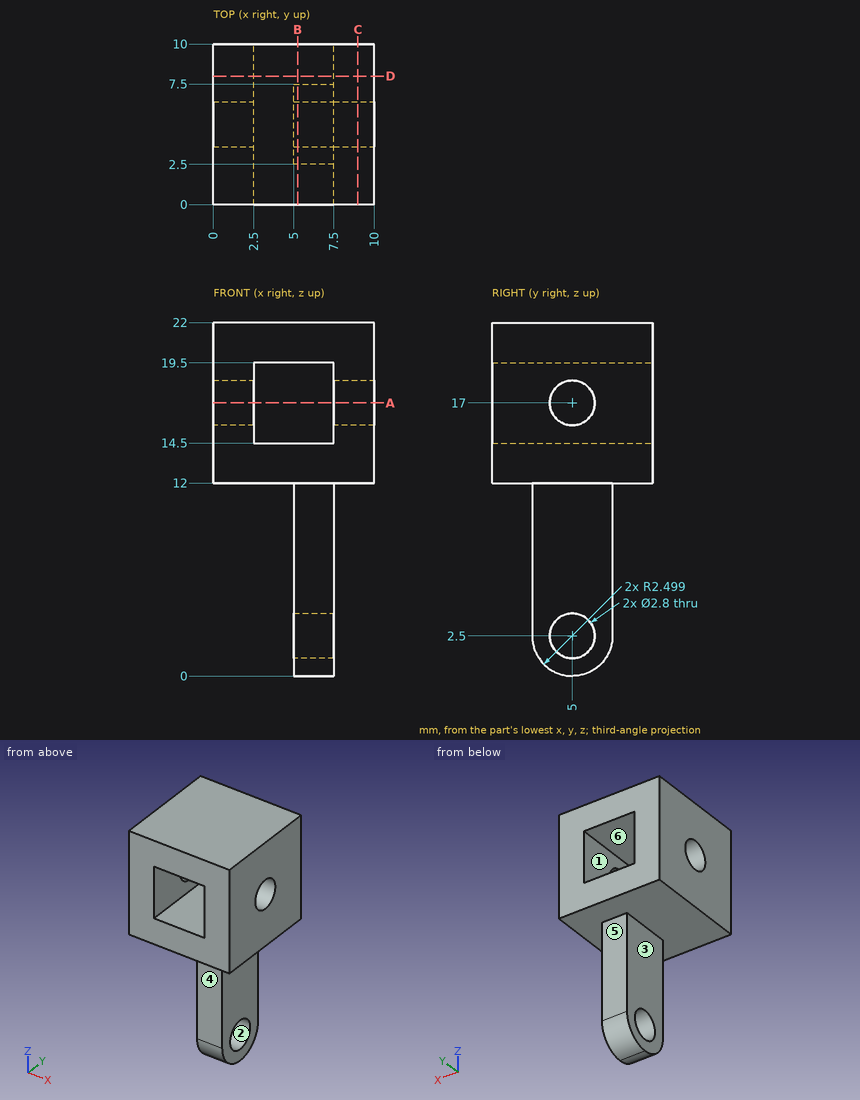
Geometry: see drawing. Coordinates: mm, zero at the bounding-box minimum. A direction names the side the tool comes from. Coordinates: 2 decimals unless noted, no trailing zeros. Loops run counter-clockwise (first coordinate to the right, second up) from the corner with the lowest first, then second, coordinate; pieces in that order, holes last.
(1) Section C-C on x = 9. Return the cut outline in (y, z).
(2) Section D-D on y = 8. Return the cut outline in (x, z).
(3) Material intervals for probe 1 along Y at (x, z) = (1.3, 17); probe 2 along Z at (x, y) = (4, 6.5); probe 3 along X at (y, z) = (5, 15.25), sorted ascending.
(4) Pull-direction query (X, two-part tool) for the marked faces 1, 2 and 3; classes: released by +X, released by -X, zero draft, split by the parting line, or undercut.
(5) Set-up query: the marked faces 4, 5 and 6. Return all of +Z, -Z, +X, -X, +Y, -Y with unobstructed straight access to the full face (end or side cutting, diameter ignored); none if empty.
(6) Section B-B on x = 5.25. Count the separate pieces of the cut face and the enclosed holes in it, then the cut area to 3 significant figures.
(7) First-contact query: pin 1 Ø3 at (x, z) = (2.5, 4) entering from -Y; pin 2 Ø1 at (y, z) = (7.5, 2.5) entering from +X; pin 3 Ø2.5 at (y, z) = (6, 3) entering from -X; pin 4 Ø1.2 at (x, z) = (6, 9) entering from +Y. Flat tips, straight axial feed; report the tip coordinate or a pass-through.
(8) Section A-A on z = 17. Return the cut outline in (x, y), then the cut area to 3 significant figures.
Data:
1. outline: (0, 12) - (10, 12) - (10, 22) - (0, 22) - close; hole circle Ø2.8 at (5, 17)
2. outline: (0, 12) - (10, 12) - (10, 22) - (0, 22) - close; hole (2.5, 14.5) - (7.5, 14.5) - (7.5, 19.5) - (2.5, 19.5) - close
3. probe 1: y = 0 to 3.6, 6.4 to 10
3. probe 2: z = 12 to 14.5, 19.5 to 22
3. probe 3: x = 0 to 2.5, 7.5 to 10
4. face 1: undercut
4. face 2: zero draft
4. face 3: released by -X
5. face 4: -Z, +X, -X, -Y
5. face 5: -Z, +X, -X, +Y
5. face 6: +Y, -Y
6. separate pieces: 2
6. enclosed holes: 1
6. area: 101 mm2
7. pin 1: passes through
7. pin 2: stops at x = 7.5
7. pin 3: stops at x = 5
7. pin 4: stops at y = 7.5
8. outline: (0, 0) - (2.5, 0) - (2.5, 3.6) - (0, 3.6) - close; (0, 6.4) - (2.5, 6.4) - (2.5, 10) - (0, 10) - close; (7.5, 0) - (10, 0) - (10, 3.6) - (7.5, 3.6) - close; (7.5, 6.4) - (10, 6.4) - (10, 10) - (7.5, 10) - close
8. area: 36.0 mm2
